Design review of the part shown in the three views and the two pictorial views. Dimensions are in mm from the part's minimum x, y and z. Coordinates: 2 decimals unless noted, no trailing zeros. Write each loop counter-clockwise with the first axis right and the second up, starting at its lowest first coordinate (ties: lowest second). Pieces come first, ordered by that corner, then holes. Notation, with made-up numbers: (48.5, -3) -> (55.5, -3) arc R14 ccw to (55.5, 11) -> close; hole circle Ø5 at (-22.75, 36). An arc over 180 degrees is marked (long way). Write each question's results on one line, items separated by ' | '.
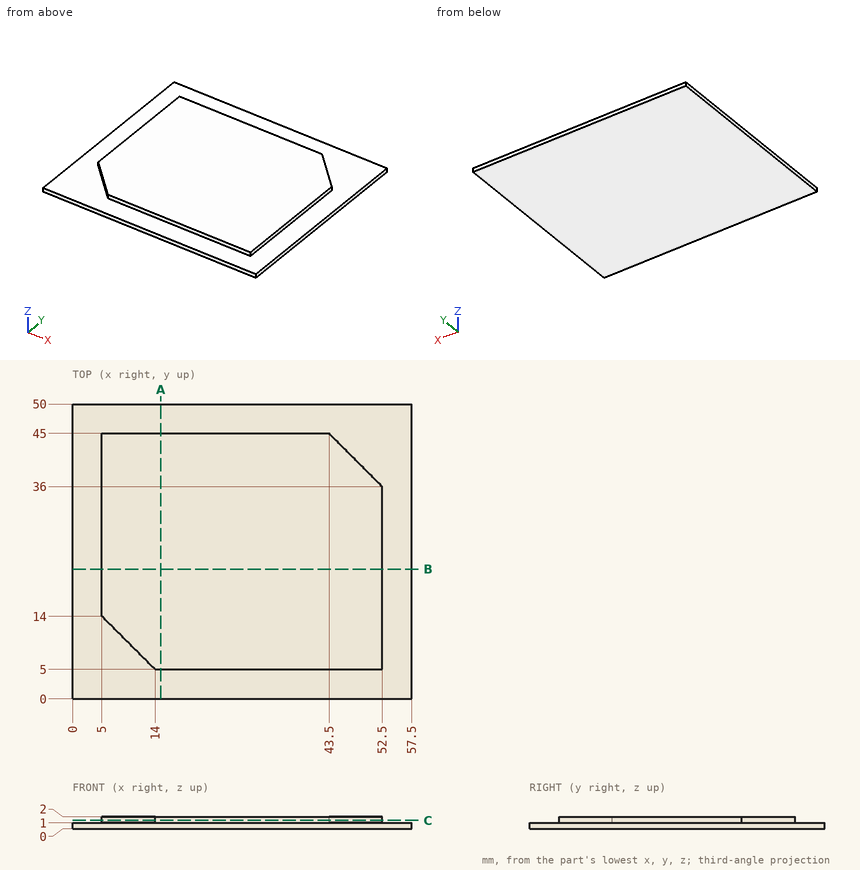
Q1. Add section B-B (y = 22). Write out the cut boundary in (x, z), plus the area to 3 significant figures.
Solution:
outline: (0, 0) -> (57.5, 0) -> (57.5, 1) -> (52.5, 1) -> (52.5, 2) -> (5, 2) -> (5, 1) -> (0, 1) -> close | area: 105 mm²
Q2. Add section C-C (z = 1.4). Write out the cut boundary in (x, y), plus the area to 3 significant figures.
Solution:
outline: (5, 14) -> (14, 5) -> (52.5, 5) -> (52.5, 36) -> (43.5, 45) -> (5, 45) -> close | area: 1,820 mm²
Q3. Clearance check with flat-ended pins moving along their axes: P1, Ø0.5, axis at y = 16.5, z = 1.5, coming from the +X side; P2, Ø0.5, axis at x = 26, z = 1.5, coming from the +Y side; P3, Ø0.5, axis at x = 35, z = 1.5, coming from the -Y side. State where each tip first meets the part, or that it passes through.
Solution:
P1: x = 52.5 | P2: y = 45 | P3: y = 5
Q4. Add section A-A (x = 15). Write out the cut boundary in (y, z).
Solution:
outline: (0, 0) -> (50, 0) -> (50, 1) -> (45, 1) -> (45, 2) -> (5, 2) -> (5, 1) -> (0, 1) -> close
Q5. For line 1 (Y direction, x = 17.5, z = 1.75); line 2 (X direction, y = 17.5, z = 1.5); line 3 (Z direction, x = 6, y = 3), list the stretches that pass through material, from the lowest coordinate up. Write a range as from..to.
Solution:
line 1: 5..45 | line 2: 5..52.5 | line 3: 0..1
